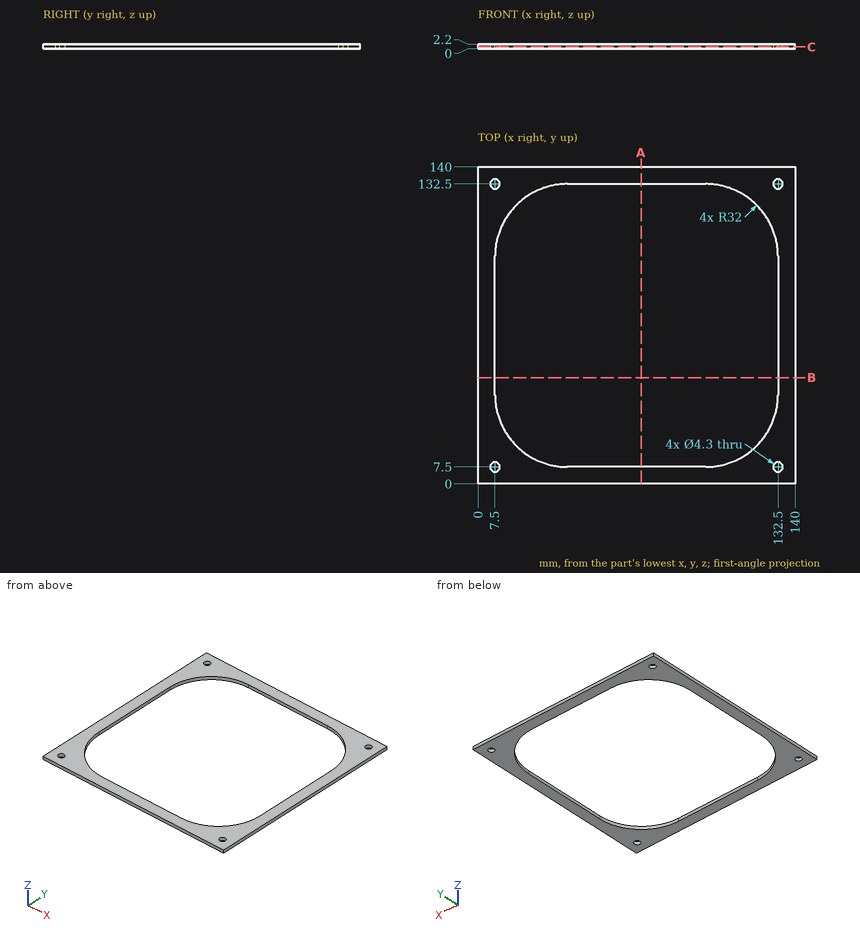
Here's the drawing with two shaded views (mm, measured from the low corner). I have some questions. Round coordinates to 2 decimals unless told otherwise and drop trailing zeros. Loops run counter-clockwise (first coordinate to the right, second up) from the corner with the lowest first, then second, coordinate; pieces in that order, holes last.
1. Suppose I cut it at C-C, the plane z = 0.9. Please give me the cut outline in (x, y), and give its area (3 significant figures).
Answers:
outline: (0, 0) - (140, 0) - (140, 140) - (0, 140) - close; hole circle Ø4.3 at (7.5, 7.5); hole circle Ø4.3 at (7.5, 132.5); hole (7.5, 39.5) arc R32 ccw to (39.5, 7.5) - (100.5, 7.5) arc R32 ccw to (132.5, 39.5) - (132.5, 100.5) arc R32 ccw to (100.5, 132.5) - (39.5, 132.5) arc R32 ccw to (7.5, 100.5) - close; hole circle Ø4.3 at (132.5, 7.5); hole circle Ø4.3 at (132.5, 132.5)
area: 4,800 mm2
2. Will this pin go through, and if not, where does the flat tip stop? pin 1 (1.1 mm diameter, centred on y = 78.5, z = 1, fed in from -X).
Answers:
pin 1: stops at x = 0
3. If I drill on probe 1 along Y at (x, z) = (99, 1.55); probe 2 along X at (y, z) = (113.5, 0.7), over which ranges is the centre line in solid material (lowest first)?
Answers:
probe 1: y = 0 to 7.5, 132.5 to 140
probe 2: x = 0 to 10.26, 129.74 to 140
4. Suppose I cut it at A-A, the plane x = 72. Please give me the cut outline in (y, z), and give its area (3 significant figures).
Answers:
outline: (0, 0) - (7.5, 0) - (7.5, 2.2) - (0, 2.2) - close; (132.5, 0) - (140, 0) - (140, 2.2) - (132.5, 2.2) - close
area: 33.0 mm2
